Here's the drawing with two shaded views (mm, measured from the low corner). I have some questions. Give positions to 0.01 mm unless a question says otherwise; leave off trailing zeros. Loops run counter-clockwise (first coordinate to the right, second up) from the corner with the lowest first, then second, coordinate; pieces in that order, holes last. Notation, with made-up numbers: (38.25, 77.5) - (82.25, 77.5) arc R12 ccw to (82.25, 100.5) - close; hole circle Ø6 at (74.25, 66.25). An arc over 180 degrees is marked (long way). Answer as a JSON object with one key per item and string values. Group by question number.
Item 1: Suppose I cut it at B-B on y = 21. Write out the boundary of the cut face in (x, z) (1 decimal), and give its area (3 significant figures).
Item 2: Suppose I cut it at C-C on x = 3.5. Write out the boundary of the cut face in (y, z).
Item 3: Please list where these lines run through material, in increasing order: L1, parallel to Z at x = 4.75, y = 20; L2, parallel to Z at x = 7, y = 21.5 (1 decimal); L3, parallel to Z at x = 3.75, y = 24.
Item 4: Suppose I cut it at A-A on z = 40. Write out the boundary of the cut face in (x, y).
Item 5: Will these pins go through, and if not, where does the flat tip stop? pin 1 (2.5 mm diameter, centred on y = 20, z = 8, fed in from +X); pin 2 (2 mm diameter, centred on x = 3, z = 52.5, fed in from +Y); pin 3 (4 mm diameter, centred on x = 1.5, y = 6.5, fed in from -Z) (1 decimal); pin 4 (4 mm diameter, centred on x = 3.5, z = 49.5, fed in from -Y).
Item 6: Suppose I cut it at D-D on y = 29.5. Write out the boundary of the cut face in (x, z) (1 decimal).
Item 7: Thinking about a two-plate mould opening in Y: for the marked faces 1, 2 and 3, which applies, pulls with the +Y half, pulls with the -Y half, needs draft (parallel to the pull), parting line crosses it, or undercut?
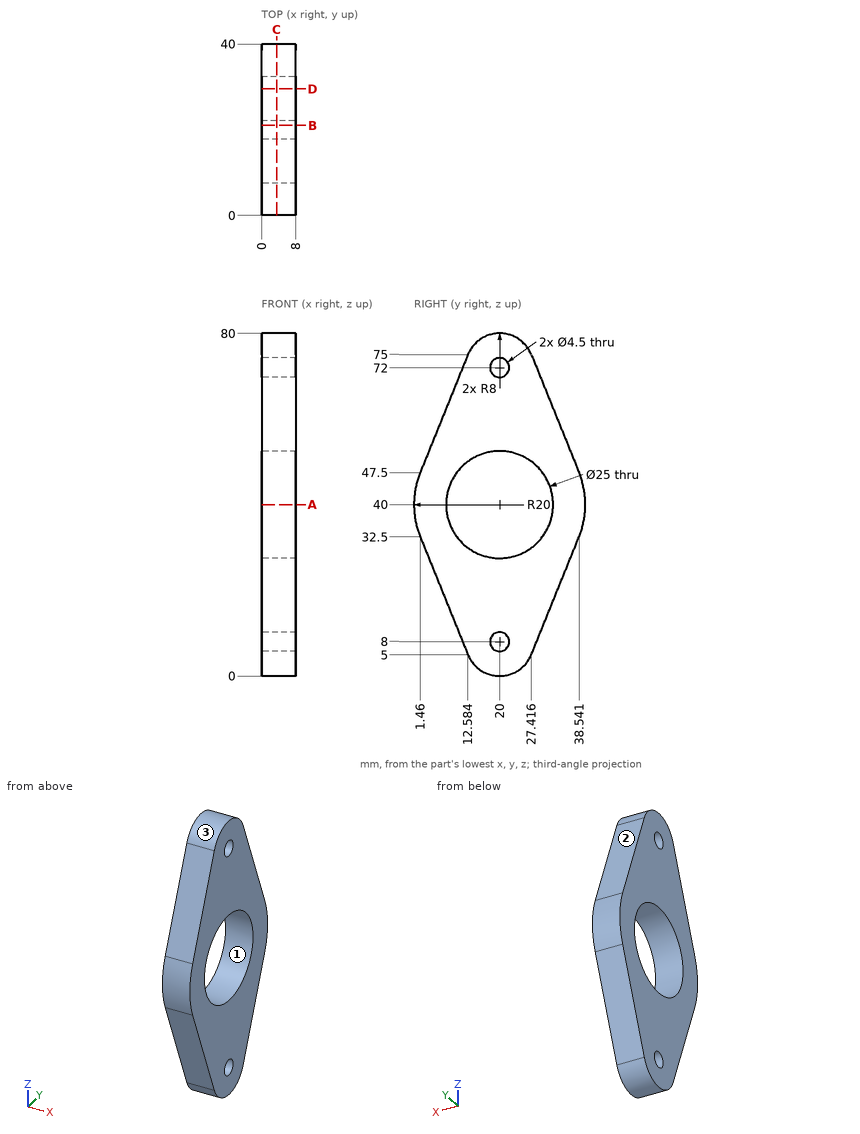
Worked out:
{
 "1": {"outline": "(0, 0.1) - (8, 0.1) - (8, 6) - (0, 6) - close; (0, 10) - (8, 10) - (8, 27.5) - (0, 27.5) - close; (0, 52.5) - (8, 52.5) - (8, 70) - (0, 70) - close; (0, 74) - (8, 74) - (8, 79.9) - (0, 79.9) - close", "area": "375 mm2"},
 "2": {"outline": "(1.46, 32.5) - (12.58, 5) arc R8 ccw to (27.42, 5) - (38.54, 32.5) arc R20 ccw to (38.54, 47.5) - (27.42, 75) arc R8 ccw to (12.58, 75) - (1.46, 47.5) arc R20 ccw to start; hole circle Ø25 at (20, 40); hole circle Ø4.5 at (20, 8); hole circle Ø4.5 at (20, 72)"},
 "3": {"L1": "z = 0 to 5.75, 10.25 to 27.5, 52.5 to 69.75, 74.25 to 80", "L2": "z = 0.1 to 6.3, 9.7 to 27.6, 52.4 to 70.3, 73.7 to 79.9", "L3": "z = 1.07 to 28.16, 51.84 to 78.93"},
 "4": {"outline": "(0, 0) - (8, 0) - (8, 7.5) - (0, 7.5) - close; (0, 32.5) - (8, 32.5) - (8, 40) - (0, 40) - close"},
 "5": {"pin 1": "passes through", "pin 2": "stops at y = 36.92", "pin 3": "stops at z = 15.1", "pin 4": "stops at y = 1.46"},
 "6": {"outline": "(0, 10.2) - (8, 10.2) - (8, 31.9) - (0, 31.9) - close; (0, 48.1) - (8, 48.1) - (8, 69.8) - (0, 69.8) - close"},
 "7": {"face 1": "undercut", "face 2": "pulls with the +Y half", "face 3": "parting line crosses it"}
}
